Source: CAD feature listing. Evaluate the final solid. Frame: model axes, mm. A direction names the side the tool comes from. Coordinates: 2 decimals unless noted, no trailing zeros. Loops run counter-clockwise (first coordinate to the right, second up) from the corner with the lowest first, then second, coordinate; pieces in that order, holes last.
Item 1: Section query C-C, the plane z = 4.75. Return the cut outline in (x, y).
Item 2: Reachability of faces 1 (the cylindrical face through (14.066, 10.648, -0.74)), 2 (the flat face through (16, 3, 0)) from +Z, -Z, +X, -X, +Y, -Y: full face, straight path, thin tool, end or side. Return the list, or none.
Item 3: Section query D-D, the plane x = -11.5. Return the cut outline in (y, z), then the cut area to 3 significant figures.
Item 4: Section query B-B, the plane x = -7. Return the cut outline in (y, z).
Item 5: Section query A-A, the plane y = 0. Return the cut outline in (x, z).
Item 6: Pin query (flat end, axial travel): pin 1 Ø2 at (y, z) = (1, 4.5) entering from +X; pin 2 Ø2 at (x, z) = (-6, 2) entering from -Y; pin 3 Ø1.5 at (x, y) = (-12.5, 13) entering from +Z. Return the tip coordinate at first contact, or that it passes through.
Item 7: Line query: probe 1 along Y at (x, z) = (0, 1.75); probe 2 along Y at (x, z) = (0, -0.7); probe 3 along X at (y, z) = (-6.5, 1). Output: solid intervals per line, ascending.
Autodesk Inventor part; units mm, degrees
ref_plane "YZ Plane" through (0, 0, 0) normal (1, 0, 0) x (0, 1, 0)
ref_plane "XZ Plane" through (0, 0, 0) normal (0, 1, 0) x (-1, 0, 0)
ref_plane "XY Plane" through (0, 0, 0) normal (0, 0, 1) x (1, 0, 0)
sketch "Sketch1" plane through (0, 0, 0) normal (0, 0, 1) x (1, 0, 0)
  circle A0 centre (0, 0) radius 10
  circle A1 centre (0, 0) radius 16
  dimension "d0" = 20
  dimension "d1" = 32
extrude "Extrusion1" add sketch "Sketch1" along normal blind 5.5
sketch "Sketch2" plane through (0, 0, 0) normal (0, 0, -1) x (-1, 0, 0)
  circle A0 centre (0, 0) radius 10
  circle A1 centre (-0.1785, 0) radius 17.5
  dimension "d4" = 20
  dimension "d5" = 35
extrude "Extrusion2" add sketch "Sketch2" along normal blind 1.5
properties part number "F6004" material "Stainless Steel"
Verdict:
1. outline: circle Ø32 at (0, 0); hole circle Ø20 at (0, 0)
2. face 1: +Z, -Z
2. face 2: +Z
3. outline: (-13.03, -1.5) - (13.03, -1.5) - (13.03, 0) - (11.12, 0) - (11.12, 5.5) - (-11.12, 5.5) - (-11.12, 0) - (-13.03, 0) - close
3. area: 161 mm2
4. outline: (-15.96, -1.5) - (-7.14, -1.5) - (-7.14, 5.5) - (-14.39, 5.5) - (-14.39, 0) - (-15.96, 0) - close; (7.14, -1.5) - (15.96, -1.5) - (15.96, 0) - (14.39, 0) - (14.39, 5.5) - (7.14, 5.5) - close
5. outline: (-17.32, -1.5) - (-10, -1.5) - (-10, 5.5) - (-16, 5.5) - (-16, 0) - (-17.32, 0) - close; (10, -1.5) - (17.68, -1.5) - (17.68, 0) - (16, 0) - (16, 5.5) - (10, 5.5) - close
6. pin 1: stops at x = 16
6. pin 2: stops at y = -15.2
6. pin 3: stops at z = 0
7. probe 1: y = -16 to -10, 10 to 16
7. probe 2: y = -17.5 to -10, 10 to 17.5
7. probe 3: x = -14.62 to -7.6, 7.6 to 14.62
